Autodesk Inventor part; units mm, degrees
ref_plane "YZ Plane" through (0, 0, 0) normal (1, 0, 0) x (0, 1, 0)
ref_plane "XZ Plane" through (0, 0, 0) normal (0, 1, 0) x (-1, 0, 0)
ref_plane "XY Plane" through (0, 0, 0) normal (0, 0, 1) x (1, 0, 0)
sketch "Sketch1" plane through (0, 0, 0) normal (0, 0, 1) x (1, 0, 0)
  line L0 (0, 0) -> (0, -1.65)
  line L1 (0, -1.65) -> (13, -1.65)
  line L2 (13, -1.65) -> (13, 0)
  line L3 (13, 0) -> (0, 0)
  dimension "d1" = 1.65
  dimension "d2" = 13
extrude "Extrusion1" add sketch "Sketch1" along normal blind 8
sketch "Sketch3" plane through (0, 0, 0) normal (0, 1, 0) x (1, 0, 0)
  line L0 (0, 0) -> (13, 0)
  line L1 (0, -8) -> (13, -8)
  line L2 (0, 0) -> (0, -8)
  line L3 (0, 0) -> (0, -3)
  line L4 (0, -8) -> (0, -5)
  line L5 (13, 0) -> (13, -3)
  line L6 (13, 0) -> (13, -8)
  line L7 (13, -8) -> (13, -5)
  line L8 (3.5, -3) -> (9.5, -3)
  line L9 (9.5, -3) -> (9.5, -5)
  line L10 (9.5, -5) -> (3.5, -5)
  line L11 (3.5, -5) -> (3.5, -3)
  dimension "d9" = 3
  dimension "d10" = 3
  dimension "d13" = 3.5
  dimension "d14" = 3.5
extrude "Extrusion2" add sketch "Sketch3" along normal blind 8 contours L8 L9 L10 L11
sketch "Sketch4" plane through (0, -1.65, 0) normal (0, -1, 0) x (1, 0, 0)
  line L0 (13, 8) -> (0, 8)
  line L1 (13, 0) -> (13, 8)
  line L2 (13, 8) -> (13, 5)
  line L3 (13, 5) -> (13, 3)
  line L4 (9.5, 5) -> (3.5, 5)
  line L5 (3.5, 5) -> (3.5, 3)
  line L6 (3.5, 5) -> (9.5, 5)
  line L7 (9.5, 5) -> (9.5, 3)
  line L8 (9.5, 3) -> (3.5, 3)
  line L9 (3.5, 3) -> (3.5, 5)
extrude "Extrusion3" add sketch "Sketch4" along normal blind 4
sketch "Sketch6" plane through (9.5, -1.65, 3) normal (0, 0, -1) x (-1, 0, 0)
  line L0 (0, -4) -> (6, -4)
  line L1 (6, -4) -> (14.5, -4)
  line L2 (14.5, -4) -> (14.5, -19)
  line L3 (14.5, -19) -> (11.5, -19)
  line L4 (11.5, -19) -> (0, -4)
  point P0 (9.5, 1.65)
  dimension "d22" = 8.5
  dimension "d23" = 15
  dimension "d24" = 3
extrude "Extrusion4" add sketch "Sketch6" against normal blind 2
sketch "Sketch7" plane through (9.5, -1.65, 3) normal (0, 0, -1) x (-1, 0, 0)
  line L0 (6, -4) -> (14.5, -4)
  line L1 (14.5, -19) -> (12.5, -19)
  line L2 (14.5, -19) -> (11.5, -19)
  line L3 (12.5, -4) -> (12.5, -6.5)
  line L4 (12.5, -19) -> (12.5, -16.5)
  circle A0 centre (12.5, -16.5) radius 0.75
  line L5 (12.5, -16.5) -> (12.5, -13.5)
  circle A1 centre (12.5, -13.5) radius 1.25
  line L6 (12.5, -13.5) -> (12.5, -10.5)
  circle A2 centre (12.5, -10.5) radius 0.75
  line L7 (12.5, -10.5) -> (12.5, -7.5)
  circle A3 centre (12.5, -7.5) radius 0.75
  point P0 (9.5, 1.65)
  dimension "d31" = 2
  dimension "d45" = 2.5
  dimension "d46" = 2.5
  dimension "d47" = 1.5
  dimension "d48" = 3
  dimension "d49" = 2.5
  dimension "d50" = 3
  dimension "d51" = 1.5
  dimension "d52" = 3
  dimension "d53" = 1.5
fillet "Fillet1" radius 2 1 edges at (3.5, -5.65, 4)
fillet "Fillet2" radius 2 2 edges at (-2, -20.65, 4) (-5, -20.65, 4)
fillet "Fillet3" radius 2 1 edges at (-5, -5.65, 4)
extrude "Extrusion6" cut sketch "Sketch7" against normal blind 2
sketch "Sketch8" plane through (9.5, -1.65, 3) normal (0, 0, -1) x (-1, 0, 0)
  line L0 (0, 1.65) -> (0, 9.65)
  line L1 (0, 1.65) -> (0, 5.65)
  line L2 (0, 9.65) -> (2, 9.65)
  line L3 (6, 9.65) -> (4, 9.65)
  line L4 (6, 9.65) -> (0, 9.65)
  line L5 (-3.5, 1.65) -> (9.5, 1.65)
  line L6 (6, 1.65) -> (6, 5.65)
  line L7 (0, 9.65) -> (2, 9.65)
  line L8 (2, 9.65) -> (0, 5.65)
  line L9 (0, 5.65) -> (0, 9.65)
  line L10 (4, 9.65) -> (6, 5.65)
  line L11 (6, 1.65) -> (6, 9.65)
  line L12 (6, 9.65) -> (6, 5.65)
  line L13 (4, 9.65) -> (6, 9.65)
  dimension "d59" = 4
  dimension "d60" = 2
  dimension "d61" = 2
extrude "Extrusion7" cut sketch "Sketch8" against normal blind 10 contours L0 L2 L8 | L10 L3 L11
properties part number "Control Horn"
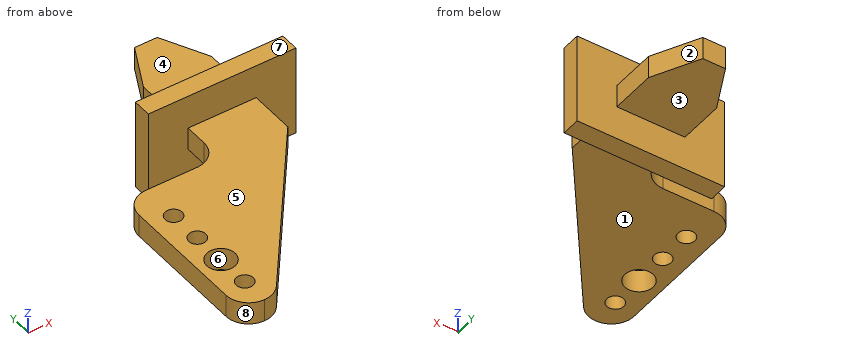
For this review, take the finished solid that the model builds, in its own axes (mm). Face numbers are marked on the shaded views. A direction names the side the tool comes from. Give positions to 0.01 mm unless a question says otherwise; leave off trailing zeros. Loops run counter-clockwise (first coordinate to the right, second up) from the corner with the lowest first, then second, coordinate; pieces in that order, holes last.
Item 1: Take a section at D-D, the plane y = -12.5. State the section outline as (x, z) points, and give its area (3 significant figures).
Item 2: Take a section at A-A, the plane z = 4.5. Give the number of separate pieces and of enclosed holes in the cut face, and give its area (3 significant figures).
Item 3: Draft analysis for pull direction X (two halves, no side actions). For the marked faces 6, 7 and 8, state which applies: +X half, -X half, draft (parallel to the pull), parting line (faces both ways), or undercut.
Item 4: Take a section at C-C, the plane x = 8. State the section outline as (y, z) points.
Item 5: Insertion check: pin 1 (3 mm diameter, centred on x = -3, y = -15.15, fed in from +Z); pin 2 (4 mm diameter, centred on x = 5, z = 4.5, fed in from -Y); pin 3 (4 mm diameter, centred on y = -17.5, z = 1.5, fed in from +X). Each pin has a flat end and moves straight along its axis. Give the tip position at first contact, or say it passes through.
Item 6: For line 1 along Y through (x, z) = (-3, 4.2); line 2 along Y through (x, z) = (10, 7.5); line 3 along Z through (x, y) = (7.5, -1.75), list the stretches that pass through material, from the lowest coordinate up.
Item 7: Take a section at B-B, the plane y = -18.15. State the section outline as (x, z) points.
Item 8: Tool access review of the marked faces 1, 2, 3, 4 and 5: name each direction out of +Z, -Z, +X, -X, +Y, -Y from which nothing blocks a thin tool from reaching the whole face with its end or side.
Calculated:
1. outline: (-5, 3) - (-3.66, 3) - (-3.66, 5) - (-5, 5) - close; (-2.34, 3) - (4.25, 3) - (4.25, 5) - (-2.34, 5) - close
1. area: 15.8 mm2
2. separate pieces: 1
2. enclosed holes: 4
2. area: 205 mm2
3. face 6: undercut
3. face 7: draft
3. face 8: -X half
4. outline: (-7.61, 3) - (-1.65, 3) - (-1.65, 0) - (0, 0) - (0, 3) - (7, 3) - (7, 5) - (0, 5) - (0, 8) - (-1.65, 8) - (-1.65, 5) - (-7.61, 5) - close
5. pin 1: stops at z = 5
5. pin 2: stops at y = -14.13
5. pin 3: stops at x = 1.43
6. line 1: y = -20.65 to -18.9, -17.4 to -16.4, -13.9 to -12.9, -11.4 to -9.9, -8.4 to -5.65
6. line 2: y = -1.65 to 0
6. line 3: z = 3 to 5
7. outline: (-5, 3) - (-3.75, 3) - (-3.75, 5) - (-5, 5) - close; (-2.25, 3) - (-0.08, 3) - (-0.08, 5) - (-2.25, 5) - close
8. face 1: -Z, +X, -X, -Y
8. face 2: +Z, -Z, +X, +Y
8. face 3: -Z, +X, -X, +Y
8. face 4: +Z, +X, -X, +Y
8. face 5: +Z, +X, -X, -Y
